Input: part model. Units: mm. Frame: model coordinates. Round coordinates to 2 decimals unless told otherwise and drop trailing zeros. Loops run counter-clockwise (first coordinate to the right, second up) from the corner with the lowest first, then second, coordinate; pieces in that order, holes last. Notation, with made-up numbers: (-22.75, 73.25) -> (-8.75, 73.25) arc R26 ccw to (-8.75, 88.25) -> close; hole circle Ø6 at (49.25, -27.5). An arc over 180 degrees is marked (long way). Answer as a JSON object with one key per item and string values. Group by question number.
Item 1: Pin query (flat end, axial travel): pin 1 (1 mm diameter, centred on x = -78.5, y = 1, fed in from -Z); pin 2 (1 mm diameter, centred on x = -82, y = 1, fed in from +Z); pin 3 (1 mm diameter, centred on x = -89, y = 1.5, fed in from -Z). Return the tip coordinate at first contact, or that it passes through.
Item 2: Section query C-C on x = -78. Return loops of the section in (y, z).
Item 3: Material intervals for line 1 (X direction, y = 1, z = 0); line 2 (Z direction, x = -76.5, y = 1.8); line 3 (Z direction, x = -28, y = 0.6), sorted ascending. Write a range as [from, to].
Item 4: Draft query along X for faces 1 (the cylindrical face through (-88.2, 0.99, 49.21)), 2 (the flat face through (-76, 0, 47)), 3 (the cylindrical face through (-90.77, 0.99, -0.33)). Return one class per face: released by +X, released by -X, zero draft, split by the parting line, or undercut.
Item 5: Section query D-D on z = 29. Return loops of the section in (x, y), and give its area (3 significant figures).
Item 6: Section query B-B on z = 0. Return loops of the section in (x, y).
Item 7: Section query A-A on y = 1.7. Return loops of the section in (x, z).
from build123d import *

# Parameters (mm, degrees)
SKETCH_1_R          = 101
SKETCH_1_R_2        = 85.5
SKETCH_1_R_3        = 2.5
EXTRUDE_2_DEPTH     = 2
SKETCH_4_R          = 2.5
CUT_EXTRUDE_2_DEPTH = 2
SKETCH_5_R          = 2.5
CUT_EXTRUDE_3_DEPTH = 2


with BuildPart() as part:
    # 草图1 → 凸台-拉伸2 (new body)
    with BuildSketch(Plane(origin=(0, 0, 0), x_dir=(1, 0, 0), z_dir=(0, 1, 0))):
        with Locations(Location((0, 0, 0), (0, 0, 270))):
            Circle(SKETCH_1_R)
        with Locations(Location((0, 0, 0), (0, 0, 270))):
            Circle(SKETCH_1_R_2, mode=Mode.SUBTRACT)
        with Locations(Location((0, 93.25, 0), (0, 0, 270))):
            Circle(SKETCH_1_R_3, mode=Mode.SUBTRACT)
        with Locations(Location((93.25, 0, 0), (0, 0, 270))):
            Circle(SKETCH_1_R_3, mode=Mode.SUBTRACT)
        with Locations(Location((0, -93.25, 0), (0, 0, 270))):
            Circle(SKETCH_1_R_3, mode=Mode.SUBTRACT)
        with Locations(Location((-93.25, 0, 0), (0, 0, 270))):
            Circle(SKETCH_1_R_3, mode=Mode.SUBTRACT)
    extrude(amount=EXTRUDE_2_DEPTH)

    # 草图4 → 切除-拉伸2 (cut)
    with BuildSketch(Plane.XZ):
        with BuildLine():
            Line((87.468565782, -50.5), (74.045172024, -42.75))
            ThreePointArc((74.045172024, -42.75), (0, -85.5), (-74.045172024, -42.75))
            Line((-74.045172024, -42.75), (-87.468565782, -50.5))
            ThreePointArc((-87.468565782, -50.5), (0, -101), (87.468565782, -50.5))
        make_face()
        with Locations((0, -93.25)):
            Circle(SKETCH_4_R, mode=Mode.SUBTRACT)
    extrude(amount=-CUT_EXTRUDE_2_DEPTH, mode=Mode.SUBTRACT)

    # 草图5 → 切除-拉伸3 (cut)
    with BuildSketch(Plane.XZ):
        with BuildLine():
            Line((0, 90.75), (0, 85.5))
            ThreePointArc((0, 85.5), (74.045172024, 42.75), (74.045172024, -42.75))
            Line((74.045172024, -42.75), (87.468565782, -50.5))
            ThreePointArc((87.468565782, -50.5), (97.558508455, -26.140723555), (101, 0))
            ThreePointArc((101, 0), (71.4177849, 71.4177849), (0, 101))
            Line((0, 101), (0, 95.75))
            ThreePointArc((0, 95.75), (1.767766953, 95.017766953), (2.5, 93.25))
            ThreePointArc((2.5, 93.25), (1.767766953, 91.482233047), (0, 90.75))
        make_face()
        with Locations((93.25, 0)):
            Circle(SKETCH_5_R, mode=Mode.SUBTRACT)
    extrude(amount=-CUT_EXTRUDE_3_DEPTH, mode=Mode.SUBTRACT)


solid = part.part
Solved:
{
 "1": {"pin 1": "z = -45.61", "pin 2": "z = 59.66", "pin 3": "z = -48.67"},
 "2": {"outline": "(0, -45.03) -> (2, -45.03) -> (2, -35.02) -> (0, -35.02) -> close; (0, 35.02) -> (2, 35.02) -> (2, 64.16) -> (0, 64.16) -> close"},
 "3": {"line 1": "[-101, -95.75], [-90.75, -85.5]", "line 2": "[-44.17, -38.18], [38.18, 65.95]", "line 3": "[80.79, 97.04]"},
 "4": {"face 1": "released by -X", "face 2": "zero draft", "face 3": "undercut"},
 "5": {"outline": "(-96.75, 0) -> (-80.43, 0) -> (-80.43, 2) -> (-96.75, 2) -> close", "area": "32.6 mm²"},
 "6": {"outline": "(-101, 0) -> (-95.75, 0) -> (-95.75, 2) -> (-101, 2) -> close; (-90.75, 0) -> (-85.5, 0) -> (-85.5, 2) -> (-90.75, 2) -> close"},
 "7": {"outline": "(-87.47, -50.5) -> (-74.05, -42.75) arc R85.5 cw to (0, 85.5) -> (0, 90.75) arc R2.5 cw to (0, 95.75) -> (0, 101) arc R101 ccw to start; hole circle Ø5 at (-93.25, 0)"}
}
